Design review of the part shown in the three views and the two pictorial views. Dimensions are in mm from the part's minimum x, y and z. Give positions to 0.01 mm unless a question says otherwise; leave off trailing zeros. Order: outer loops, then holes, each group sorted by start corner. A loop starts at its lowest first (then second) coordinate and runs counter-clockwise, first axis right, second up.
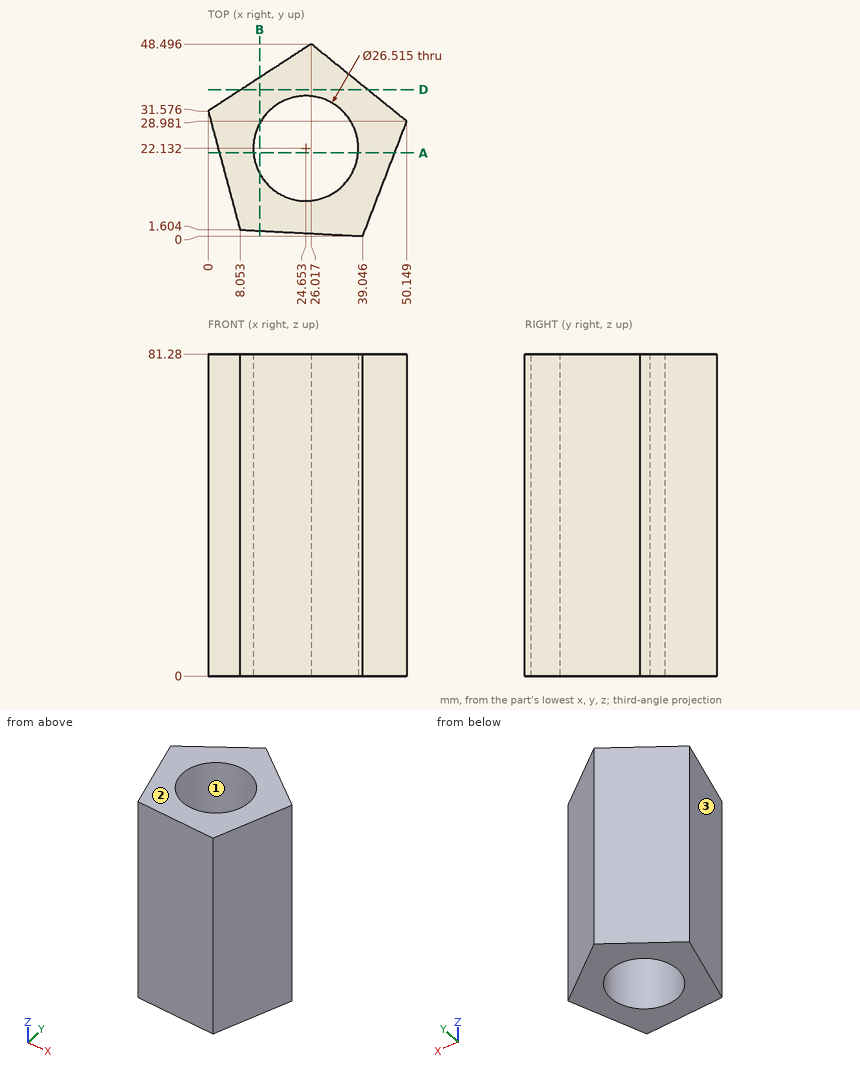
Item 1: Draft analysis for pull direction X (two halves, no side actions). For the marked faces 1, 2 and 3, state which applies: released by +X, released by -X, zero draft, split by the parting line, or undercut.
Values found:
face 1: undercut
face 2: zero draft
face 3: released by -X
Item 2: Clearance check with flat-ended pins moving along their axes: pin 1 Ø1.5 at (x, y) = (17, 35.5) entering from -Z; pin 2 Ø2 at (y, z) = (13.5, 11.5) entering from -X; pin 3 Ø10 at (x, z) = (19, 19) entering from -Y; pin 4 Ø3 at (y, z) = (13.5, 43) entering from +X. State where each tip first meets the part, or that it passes through.
Values found:
pin 1: stops at z = 0
pin 2: stops at x = 4.59
pin 3: stops at y = 0.78
pin 4: stops at x = 44.79
Item 3: Take a section at D-D (y = 37). Give the boundary of the cut face in (x, z).
Values found:
outline: (8.34, 0) - (40.23, 0) - (40.23, 81.28) - (8.34, 81.28) - close
Item 4: Take a section at B-B (x = 13). Give the boundary of the cut face in (y, z), and give its area (3 significant figures).
Values found:
outline: (1.35, 0) - (15.81, 0) - (15.81, 81.28) - (1.35, 81.28) - close; (28.45, 0) - (40.03, 0) - (40.03, 81.28) - (28.45, 81.28) - close
area: 2,120 mm2
Item 5: For line 1 (X direction, y = 33, z = 29.5) (1 decimal); line 2 (Y direction, x = 20, z = 66.5) (1 decimal); line 3 (Y direction, x = 18, z = 30) (1 decimal), list the stretches that pass through material, from the lowest coordinate up.
Values found:
line 1: x = 2.2 to 17.1, 32.2 to 45.2
line 2: y = 1 to 9.7, 34.5 to 44.6
line 3: y = 1.1 to 10.7, 33.6 to 43.3
Item 6: Take a section at A-A (y = 21). Give the boundary of the cut face in (x, z) (1 decimal), and give its area (3 significant figures).
Values found:
outline: (2.8, 0) - (11.4, 0) - (11.4, 81.3) - (2.8, 81.3) - close; (37.9, 0) - (47.1, 0) - (47.1, 81.3) - (37.9, 81.3) - close
area: 1,450 mm2
